from build123d import *

# Parameters (mm, degrees)
BOSS_EXTRUDE1_DEPTH       = 12.7
SKETCH2_R                 = 5.635000033
HAPTIC_MOTOR_CUTOUT_DEPTH = 9.557999934
SKETCH3_W                 = 5.08
SKETCH3_H                 = 6.35
HAPTIC_WIRE_CUTOUT_DEPTH  = 13.7
SKETCH4_W                 = 6.096
SKETCH4_H                 = 2.54
PINS_DEPTH                = 5.08


with BuildPart() as part:
    # Sketch1 → Boss-Extrude1 (new body)
    with BuildSketch(Plane(origin=(0, 0, 0), x_dir=(1, 0, 0), z_dir=(0, 1, 0))):
        Polygon((0, 0), (19.05, 0), (19.05, 19.05), (19.05, 38.1), (0, 38.1), (0, 19.05), align=None)
    extrude(amount=BOSS_EXTRUDE1_DEPTH)

    # Sketch2 → Haptic Motor Cutout (cut)
    with BuildSketch(Plane.XZ.offset(-12.7)):
        with Locations((8.89, -19.05)):
            Circle(SKETCH2_R)
    extrude(amount=HAPTIC_MOTOR_CUTOUT_DEPTH, mode=Mode.SUBTRACT)

    # Sketch3 → Haptic Wire Cutout (cut, through all)
    with BuildSketch(Plane.XZ):
        with Locations((8.89, -27.255072104)):
            Rectangle(SKETCH3_W, SKETCH3_H)
    extrude(amount=-HAPTIC_WIRE_CUTOUT_DEPTH, mode=Mode.SUBTRACT)

    # Sketch4 → Pins (add)
    with BuildSketch(Plane.XZ):
        with Locations((10.668, -35.56)):
            Rectangle(SKETCH4_W, SKETCH4_H)
    pins = extrude(amount=PINS_DEPTH)

    # Mirror1: Pins across plane
    add(pins.mirror(Plane(origin=(0, 0, -19.05), x_dir=(1, 0, 0), z_dir=(0, 0, -1))))


solid = part.part
Could you check a few things on this model? Use its own coordinates, in mm. A direction names the side the tool comes from. Give positions to 0.01 mm unless a question says otherwise; leave off trailing zeros. Order: outer loops, then holes, each group sorted by start corner. A loop starts at its lowest first (then second) coordinate and runs counter-clockwise, first axis right, second up. Notation, with made-up numbers: (-20.5, 22) - (-6.5, 22) arc R4 cw to (-6.5, 26) - close; hole circle Ø3 at (20.25, -6). An arc over 180 degrees is marked (long way). Return JSON: item names as keys, results as strings. Group by question number.
Q1. Suppose I cut it at C-C, the plane z = -19.05. Please give me the cut outline in (x, y) (3 decimals), and give its area (3 significant figures).
Q2. Thinking about a two-plate mould opening in Z: for faces 1 (the face through (11, -3, -36.83)), 2 (the face through (9, 3.142, -19)), 3 (the face through (13.716, -3, -3)), which applies, pulls with the +Z half, pulls with the -Z half, needs draft (parallel to the pull), parting line crosses it, or undercut?
Q3. Will these pins go through, and if not, where does the flat tip stop? pin 1 Ø1.3 at (y, z) = (-3, -36) entering from +X; pin 2 Ø2.5 at (x, y) = (12, -3.5) entering from +Z; pin 3 Ø2 at (y, z) = (-3.5, -3) entering from -X.
Q4. Suppose I cut it at A-A, the plane y = -2.75. Please give me the cut outline in (x, z).
Q5. Suppose I cut it at D-D, the plane y = 7.5. Please give me the cut outline in (x, z) (3 decimals), and give its area (3 significant figures).
Q6. Which directions (+Z, -Z, +X, -X, +Y, -Y) give clear straight access to the entire face, cutting with the end or side of a thin tool? Please do faces 4 (the face through (11.43, 6, -27)), 5 (the face through (9.1, 7.99, -13.42)), 6 (the face through (11, -3, -34.29)).
Q7. Suppose I cut it at B-B, the plane x = 8.75. Please give me the cut outline in (y, z).
Q8. Please list where these lines run through material, in increasing order: line 1 along X through (y, z) = (4.25, -26); line 2 along X through (y, z) = (10, -19.05) (3 decimals); line 3 along Z through (x, y) = (8.89, 10.25) (3 decimals). Write a range as [from, to].
Resolved:
{
 "1": {"outline": "(0, 0) - (19.05, 0) - (19.05, 12.7) - (14.525, 12.7) - (14.525, 3.142) - (3.255, 3.142) - (3.255, 12.7) - (0, 12.7) - close", "area": "134 mm2"},
 "2": {"face 1": "pulls with the -Z half", "face 2": "undercut", "face 3": "needs draft"},
 "3": {"pin 1": "stops at x = 13.72", "pin 2": "stops at z = -1.27", "pin 3": "stops at x = 7.62"},
 "4": {"outline": "(7.62, -36.83) - (13.72, -36.83) - (13.72, -34.29) - (7.62, -34.29) - close; (7.62, -3.81) - (13.72, -3.81) - (13.72, -1.27) - (7.62, -1.27) - close"},
 "5": {"outline": "(0, -38.1) - (19.05, -38.1) - (19.05, 0) - (0, 0) - close; hole (6.35, -30.43) - (11.43, -30.43) - (11.43, -24.08) arc R5.635 ccw (long way) to (6.35, -24.08) - close", "area": "596 mm2"},
 "6": {"face 4": "+Y, -Y", "face 5": "+Y", "face 6": "+X, -X, -Y"},
 "7": {"outline": "(-5.08, -36.83) - (0, -36.83) - (0, -38.1) - (12.7, -38.1) - (12.7, -30.43) - (0, -30.43) - (0, -34.29) - (-5.08, -34.29) - close; (-5.08, -3.81) - (0, -3.81) - (0, -24.08) - (3.14, -24.08) - (3.14, -13.42) - (12.7, -13.42) - (12.7, 0) - (0, 0) - (0, -1.27) - (-5.08, -1.27) - close"},
 "8": {"line 1": "x = [0, 6.35], [11.43, 19.05]", "line 2": "x = [0, 3.255], [14.525, 19.05]", "line 3": "z = [-38.1, -30.43], [-13.415, 0]"}
}
